CAD build for the part. Positions are in the model's coordinates, mm. Face numbers are marked on the shaded views. A direction names the side the tool comes from. Round coordinates to 2 decimals unless told otherwise and drop trailing zeros. Write each loop counter-clockwise with the first axis right and the second up, starting at its lowest first coordinate (ties: lowest second). Pieces come first, ordered by that corner, then holes. Notation, with made-up numbers: (-29.5, 5.5) - (10.5, 5.5) arc R17 cw to (10.5, 29.5) - close; hole circle Ø4 at (-6, 27). An arc over 180 degrees is marked (long way). Use one line per item in the form item = value. Start each with the question number.
Item 1: Band-saw the part on D-D, the plane x = 0.25. List the corners of the cut face in (y, z), and give its area (3 significant figures).
Item 2: Pull direction Z, two halves, no side cores. Call the marked faces 4, 5, 6 and 7: +Z half, -Z half, draft (parallel to the pull), parting line (faces both ways), or undercut.
Item 3: Drill centre lines: L1, parallel to Y at x = 6.5, z = -11.5; L2, parallel to X at y = -7, z = 4; L3, parallel to Z at x = 6, y = -4.75. Where is each one in solid material? Low to high.
Item 4: Pin check, flat tips, straight feed: pin 1 (12 mm diameter, centred on x = 6.5, z = 0, fed in from -Y); pin 2 (9 mm diameter, centred on y = 4, z = 17, fed in from +X); pin 3 (3 mm diameter, centred on y = -5, z = -9, fed in from +X); pin 4 (4 mm diameter, centred on x = 14.5, y = 2.5, fed in from -Z). Stop position of each tip, or through.
Item 5: Tool access for the marked faces 1, 2 and 3: list every direction of +Z, -Z, +X, -X, +Y, -Y with a clear straight run to the whole face (end or side of a thin tool).
Item 6: Band-saw the part on A-A, the plane y = -3.75. List the corners of the cut face in (x, z), and give its area (3 significant figures).
Item 7: Band-saw the part on C-C, the plane x = 7. List the corners of the cut face in (y, z), and give its area (3 significant figures).
Item 8: Band-saw the part on B-B, the plane z = 0.5. List the corners of the cut face in (x, y), and give its area (3 significant figures).
from build123d import *

# Parameters (mm, degrees)
F0_W        = 12.5
F0_H        = 18
F0_W_2      = 9.62
F0_H_2      = 15.12
F1_DEPTH    = 30
F1_FACE_W   = 12.5
F1_FACE_H   = 18
F1_FACE_W_2 = 9.62
F1_FACE_H_2 = 15.12
F2_ANGLE    = 65
F3_DEPTH    = 15


with BuildPart() as f1:
    # F0 (on Top) → F1 (new body)
    with BuildSketch(Plane.XY):
        Rectangle(F0_W, F0_H)
        Rectangle(F0_W_2, F0_H_2, mode=Mode.SUBTRACT)
    extrude(amount=F1_DEPTH)

    # F1_face (on face) → F2 (revolve)
    with BuildSketch(Plane(origin=(0, 0, 0), x_dir=(1, 0, 0), z_dir=(0, 0, -1))):
        Rectangle(F1_FACE_W, F1_FACE_H)
        Rectangle(F1_FACE_W_2, F1_FACE_H_2, mode=Mode.SUBTRACT)
    revolve(axis=Axis((6.25, 0, 0), (0, -1, 0)), revolution_arc=F2_ANGLE)

    # F3 (add): a face of the model
    f3_faces = [f1.faces().sort_by_distance(p)[0] for p in [
        (3.6086358641, -8.78085393, -5.664423669),
    ]]
    extrude(f3_faces, amount=F3_DEPTH)


solid = f1.part
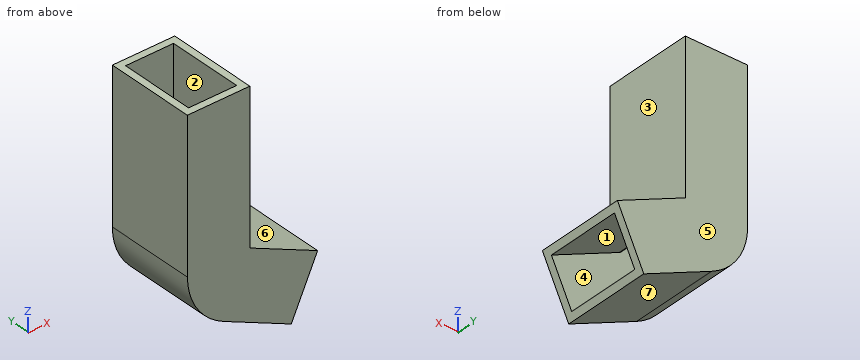
Determined:
q1.outline = (-9, -10.97) - (9, -10.97) - (9, 30) - (7.56, 30) - (7.56, -9.29) - (-7.56, -9.29) - (-7.56, 30) - (-9, 30) - close
q1.area = 143 mm²
q2.face_4 = undercut
q2.face_5 = draft
q2.face_6 = +Z half
q2.face_7 = -Z half
q3.L1 = -9 to -7.56, 7.56 to 9
q3.L2 = -6.25 to -4.81, 4.81 to 6.25
q3.L3 = -13.68 to -12.09, -1.47 to 30
q4.pin_1 = -9
q4.pin_2 = 6.25
q4.pin_3 = 19.3
q4.pin_4 = -17.67
q5.face_1 = none
q5.face_2 = +Z
q5.face_3 = +Z, +X, +Y, -Y
q6.outline = (-6.25, 0) arc R12.5 ccw to (0.97, -11.33) - (14.56, -17.67) - (15.17, -16.36) - (1.58, -10.02) arc R11.06 cw to (-4.81, 0) - (-4.81, 30) - (-6.25, 30) - close; (4.81, 0) arc R1.44 ccw to (5.64, -1.31) - (19.24, -7.64) - (19.84, -6.34) - (6.25, 0) - (6.25, 30) - (4.81, 30) - close
q6.area = 150 mm²
q7.outline = (-9, -14.14) - (9, -14.14) - (9, -0.35) - (-9, -0.35) - close; hole (-7.56, -12.55) - (7.56, -12.55) - (7.56, -1.94) - (-7.56, -1.94) - close
q7.area = 87.8 mm²
q8.outline = (-6.25, -9) - (6.25, -9) - (6.25, 9) - (-6.25, 9) - close; hole (-4.81, -7.56) - (4.81, -7.56) - (4.81, 7.56) - (-4.81, 7.56) - close
q8.area = 79.5 mm²
